Source: CAD feature listing. Evaluate the final solid. Frame: model axes, mm. A direction names the side the tool comes from. Round coordinates to 2 decimals unless told otherwise and drop trailing zeros. Loops run counter-clockwise (first coordinate to the right, second up) from the corner with the lowest first, then second, coordinate; pieces in that order, holes last.
(1) Section C-C, the plane x = -10. Return the cut outline in (y, z).
(2) Set-up query: faces 1 (the cylindrical face through (-14.43, 7.1, 12.9)), 2 (the flat face through (2, 13, -2)). Return all of +Z, -Z, +X, -X, +Y, -Y with unobstructed straight access to the full face (end or side cutting, diameter ignored); none if empty.
(3) Section A-A, the plane z = -10. Return the cut outline in (x, y), plus the area to 3 significant figures.
(4) First-contact query: pin 1 Ø3.5 at (x, z) = (10, -10) entering from +Y; pin 2 Ø5 at (x, z) = (-4, 2.5) entering from +Y. Flat tips, straight axial feed; report the tip coordinate or a pass-through.
(5) Material intervals for probe 1 along Z at (x, y) = (10, 8); probe 2 along X at (y, z) = (6.75, 10); probe 3 along X at (y, z) = (5.5, 9.5), sorted ascending.
(6) Mould query, pull axis X, two halves, no side actions, for faces 3 (the cylindrical face through (14.4, 7.1, 12.93)), 4 (the cylindrical face through (-11.27, 6.9, 10.97)), 5 (the cylindrical face through (-14.43, 7.1, -12.9)), 6 (the cylindrical face through (8.73, 6.9, 10.97)). Classes: pulls with the +X half, pulls with the -X half, needs draft (parallel to the pull), parting line crosses it, or undercut.
(7) Section D-D, the plane y = 1.25. Return the cut outline in (x, z).
(8) Section B-B, the plane z = 0. Return the cut outline in (x, y), plus the area to 3 significant figures.
```python
from build123d import *

# Parameters (mm, degrees)
SKETCH_1_W          = 30
SKETCH_1_H          = 27
SKETCH_1_R          = 1.6
EXTRUDE_1_DEPTH     = 14
SKETCH_2_R          = 2.5
CUT_EXTRUDE_1_DEPTH = 15
SKETCH_3_R          = 8
CUT_EXTRUDE_2_DEPTH = 1
FILLET_1_R          = 2


with BuildPart() as part:
    # 草图1 → 凸台-拉伸1 (new body)
    with BuildSketch(Plane(origin=(0, 0, 0), x_dir=(1, 0, 0), z_dir=(0, 1, 0))):
        Rectangle(SKETCH_1_W, SKETCH_1_H)
        with Locations((-10, 10)):
            Circle(SKETCH_1_R, mode=Mode.SUBTRACT)
        with Locations((10, 10)):
            Circle(SKETCH_1_R, mode=Mode.SUBTRACT)
        with Locations((10, -10)):
            Circle(SKETCH_1_R, mode=Mode.SUBTRACT)
        with Locations((-10, -10)):
            Circle(SKETCH_1_R, mode=Mode.SUBTRACT)
    extrude(amount=EXTRUDE_1_DEPTH)

    # 草图2 → 切除-拉伸1 (cut, through all)
    with BuildSketch(Plane(origin=(0, 14, 0), x_dir=(1, 0, 0), z_dir=(0, 1, 0))):
        Circle(SKETCH_2_R)
    extrude(amount=-CUT_EXTRUDE_1_DEPTH, mode=Mode.SUBTRACT)

    # 草图3 → 切除-拉伸2 (cut)
    with BuildSketch(Plane(origin=(0, 14, 0), x_dir=(1, 0, 0), z_dir=(0, 1, 0))):
        Circle(SKETCH_3_R)
    extrude(amount=-CUT_EXTRUDE_2_DEPTH, mode=Mode.SUBTRACT)

    # 圆角1
    fillet_1_edges = [part.edges().sort_by_distance(p)[0] for p in [
        (15, 7, 13.5),
        (-15, 7, 13.5),
        (-15, 7, -13.5),
        (15, 7, -13.5),
    ]]
    fillet(fillet_1_edges, radius=FILLET_1_R)


solid = part.part
```
Output values:
1. outline: (0, -13.5) - (14, -13.5) - (14, -11.6) - (0, -11.6) - close; (0, -8.4) - (14, -8.4) - (14, 8.4) - (0, 8.4) - close; (0, 11.6) - (14, 11.6) - (14, 13.5) - (0, 13.5) - close
2. face 1: +Z, -X, +Y, -Y
2. face 2: +Y
3. outline: (-15, 0) - (-11.6, 0) - (-11.6, 14) - (-15, 14) - close; (-8.4, 0) - (8.4, 0) - (8.4, 14) - (-8.4, 14) - close; (11.6, 0) - (15, 0) - (15, 14) - (11.6, 14) - close
3. area: 330 mm2
4. pin 1: stops at y = 14
4. pin 2: stops at y = 13
5. probe 1: z = -13.5 to -11.6, -8.4 to 8.4, 11.6 to 13.5
5. probe 2: x = -15 to -11.6, -8.4 to 8.4, 11.6 to 15
5. probe 3: x = -15 to -11.52, -8.48 to 8.48, 11.52 to 15
6. face 3: pulls with the +X half
6. face 4: undercut
6. face 5: pulls with the -X half
6. face 6: undercut
7. outline: (-15, -11.5) arc R2 ccw to (-13, -13.5) - (13, -13.5) arc R2 ccw to (15, -11.5) - (15, 11.5) arc R2 ccw to (13, 13.5) - (-13, 13.5) arc R2 ccw to (-15, 11.5) - close; hole circle Ø3.2 at (-10, -10); hole circle Ø3.2 at (-10, 10); hole circle Ø5 at (0, 0); hole circle Ø3.2 at (10, -10); hole circle Ø3.2 at (10, 10)
8. outline: (-15, 0) - (-2.5, 0) - (-2.5, 13) - (-8, 13) - (-8, 14) - (-15, 14) - close; (2.5, 0) - (15, 0) - (15, 14) - (8, 14) - (8, 13) - (2.5, 13) - close
8. area: 339 mm2
